from build123d import *

# Parameters (mm, degrees)
F0_R      = 12.805228
F1_DEPTH  = 13.462
F2_R      = 2.775496
F3_DEPTH  = 71.628
F4_DEPTH  = 25.4
F5_DEPTH  = 25.4
F7_DEPTH  = 65.024
F8_R      = 11.544918
F8_R_2    = 5.557541
F8_R_3    = 8.380392
F8_R_4    = 9.320439
F8_R_5    = 10.745749
F8_R_6    = 2.177584
F8_R_7    = 5.592023
F8_R_8    = 5.45278
F8_R_9    = 2.581521
F8_R_10   = 2.292272
F8_R_11   = 6.096395
F8_R_12   = 5.062779
F8_R_13   = 2.606224
F8_R_14   = 5.024667
F8_R_15   = 1.825412
F8_R_16   = 5.73906
F8_R_17   = 5.381808
F8_R_18   = 3.280323
F8_R_19   = 4.310801
F8_R_20   = 2.82533
F8_R_21   = 6.868943
F8_R_22   = 3.579928
F8_R_23   = 2.581522
F8_R_24   = 4.081744
F8_R_25   = 4.869226
F8_R_26   = 2.95209
F8_R_27   = 2.177582
F8_R_28   = 2.726392
F8_R_29   = 1.789965
F8_R_30   = 2.087438
F8_R_31   = 11.06868
F8_R_32   = 2.952267
F9_DEPTH  = 12.954
F10_W     = 19.802404
F10_H     = 13.06525
F10_W_2   = 20.198451
F10_H_2   = 12.933277
F11_DEPTH = 4.064
F13_DEPTH = 5.842


with BuildPart() as f1:
    # F0 (on Right) → F1 (new body)
    with BuildSketch(Plane.YZ):
        Polygon((-62.617041, 14.065981), (-45.4152, 25.146002), (0, 50.444398), (45.4152, 25.146002), (62.617041, 14.065981), (53.866774, 27.880948), (0, 60.095742), (-53.866774, 27.880948), align=None)
        Polygon((0, 50.444398), (-45.4152, 25.146002), (-45.4152, -55.321198), (45.415204, -55.321198), (45.4152, 25.146002), align=None)
        with Locations((0, 6.2484)):
            Circle(F0_R, mode=Mode.SUBTRACT)
    extrude(amount=F1_DEPTH)

    # F2 (on Right) → F3 (join)
    with BuildSketch(Plane.YZ):
        with Locations((0, -32.101408)):
            Circle(F2_R)
    extrude(amount=F3_DEPTH)

    # F0 (on Right) → F4 (join)
    with BuildSketch(Plane.YZ):
        Polygon((-62.617041, 14.065981), (-45.4152, 25.146002), (0, 50.444398), (45.4152, 25.146002), (62.617041, 14.065981), (53.866774, 27.880948), (0, 60.095742), (-53.866774, 27.880948), align=None)
        Polygon((0, 50.444398), (-45.4152, 25.146002), (-45.4152, -55.321198), (45.415204, -55.321198), (45.4152, 25.146002), align=None)
        with Locations((0, 6.2484)):
            Circle(F0_R, mode=Mode.SUBTRACT)
    extrude(amount=F4_DEPTH)

    # F0 (on Right) → F5 (join)
    with BuildSketch(Plane.YZ):
        Polygon((-62.617041, 14.065981), (-45.4152, 25.146002), (0, 50.444398), (45.4152, 25.146002), (62.617041, 14.065981), (53.866774, 27.880948), (0, 60.095742), (-53.866774, 27.880948), align=None)
        Polygon((0, 50.444398), (-45.4152, 25.146002), (-45.4152, -55.321198), (45.415204, -55.321198), (45.4152, 25.146002), align=None)
        with Locations((0, 6.2484)):
            Circle(F0_R, mode=Mode.SUBTRACT)
    extrude(amount=F5_DEPTH)

    # F6 (on face) → F7 (join)
    with BuildSketch(Plane(origin=(0, 0, 0), x_dir=(0, -1, 0), z_dir=(-1, 0, 0))):
        Polygon((53.866774, 27.880948), (0, 60.095742), (-53.866774, 27.880948), (-62.617041, 14.065981), (-45.4152, 25.146002), (-45.415204, -55.321198), (45.4152, -55.321198), (45.4152, 25.146002), (62.617041, 14.065981), align=None)
    extrude(amount=F7_DEPTH)

    # F8 (on face) → F9 (cut)
    with BuildSketch(Plane.XZ.offset(45.4152)):
        with Locations((-47.735427, -38.178124)):
            Circle(F8_R)
        with Locations((-49.167398, -12.04466)):
            Circle(F8_R_2)
        with Locations((-34.489699, -20.636484)):
            Circle(F8_R_3)
        with Locations((-37.353639, 0)):
            Circle(F8_R_4)
        with Locations((13.839315, -7.390756)):
            Circle(F8_R_5)
        with Locations((-16.23207, -18.846521)):
            Circle(F8_R_6)
        with Locations((-26.971854, -35.672177)):
            Circle(F8_R_7)
        with Locations((-3.344336, -22.068456)):
            Circle(F8_R_8)
        with Locations((6.679456, -21.35247)):
            Circle(F8_R_9)
        with Locations((6.321463, -31.376265)):
            Circle(F8_R_10)
        with Locations((16.345263, -30.302286)):
            Circle(F8_R_11)
        with Locations((12.407344, -44.621993)):
            Circle(F8_R_12)
        with Locations((20.641174, -49.63389)):
            Circle(F8_R_13)
        with Locations((-4.060321, -9.180719)):
            Circle(F8_R_14)
        with Locations((-26.613861, -8.106741)):
            Circle(F8_R_15)
        with Locations((-18.022032, -9.896705)):
            Circle(F8_R_16)
        with Locations((-16.590061, 7.644936)):
            Circle(F8_R_17)
        with Locations((0, 9.434899)):
            Circle(F8_R_18)
        with Locations((15.98727, 8.718913)):
            Circle(F8_R_19)
        with Locations((4.173508, 4.423001)):
            Circle(F8_R_6)
        with Locations((-10.86218, 0)):
            Circle(F8_R_20)
        with Locations((-56.327246, 0)):
            Circle(F8_R_21)
        with Locations((-60.623161, -10.254697)):
            Circle(F8_R_22)
        with Locations((-49.167398, -20.994477)):
            Circle(F8_R_23)
        with Locations((-57.759218, -19.562507)):
            Circle(F8_R_24)
        with Locations((-31.267766, -45.695972)):
            Circle(F8_R_25)
        with Locations((-19.812003, -26.006375)):
            Circle(F8_R_26)
        with Locations((-24.107913, -51.781844)):
            Circle(F8_R_27)
        with Locations((-60.623161, -47.12794)):
            Circle(F8_R_28)
        with Locations((-62.413126, -27.796337)):
            Circle(F8_R_29)
        with Locations((-39.501593, -50.349873)):
            Circle(F8_R_30)
        with Locations((-9.707933, -40.136304)):
            Circle(F8_R_31)
        with Locations((2.335547, -49.885787)):
            Circle(F8_R_32)
    extrude(amount=-F9_DEPTH, mode=Mode.SUBTRACT)

    # F10 (on face) → F11 (join)
    with BuildSketch(Plane(origin=(0, 45.415201, 2e-06), x_dir=(-1, 0, 0), z_dir=(0, 1, 0))):
        Polygon((41.411106, -3.204356), (-7.916423, -3.578231), (-7.916423, -37.325934), (41.411106, -37.325934), align=None)
        Polygon((-5.569554, -34.437824), (-5.569554, -22.560325), (-5.569554, -21.900464), (14.496882, -21.900464), (14.496882, -23.220185), (14.496882, -34.437824), (13.572769, -34.437824), align=None, mode=Mode.SUBTRACT)
        Polygon((17.929297, -34.701772), (17.929297, -21.504547), (37.7317, -21.768492), (37.7317, -34.701772), align=None, mode=Mode.SUBTRACT)
        with Locations((4.331648, -12.992339)):
            Rectangle(F10_W, F10_H, mode=Mode.SUBTRACT)
        with Locations((28.292554, -12.926353)):
            Rectangle(F10_W_2, F10_H_2, mode=Mode.SUBTRACT)
    extrude(amount=F11_DEPTH)

    # F12 (on face) → F13 (join)
    with BuildSketch(Plane(origin=(-65.024, 0, 0), x_dir=(0, -1, 0), z_dir=(-1, 0, 0))):
        Polygon((-43.786074, -20.438465), (2.748472, 0), (-38.219031, 30.080867), align=None)
        Polygon((3.604237, -53.453038), (3.604237, -3.573573), (-39.592647, -28.513306), align=None)
        Polygon((22.778634, -18.640616), (11.063425, -50.157975), (44.215863, -44.544963), align=None)
        Polygon((9.034589, -19.765744), (38.46338, -0.555568), (7.112485, 15.325424), align=None)
        Polygon((0, 56.749567), (-10.859401, 15.269949), (30.492702, 26.605241), align=None)
    extrude(amount=F13_DEPTH)


solid = f1.part
The model under review builds one solid part; all positions refer to its coordinate system, in mm. A direction names the side the tool comes from. Round coordinates to 2 decimals unless told otherwise and drop trailing zeros. Loops run counter-clockwise (first coordinate to the right, second up) from the corner with the lowest first, then second, coordinate; pieces in that order, holes last. Notation, with made-up numbers: M 46,19.25 L 65,19.25 A14 ccw 65,30.25 Z; hole C 7,-7 d6. An arc over 180 degrees is marked long. Answer as CSV lines item,"result".
1. For faces 4 (the face through (-61, -32.461, -10)), 5 (the face through (-19.18, -58.3, 20.88)), 6 (the face through (12.52, -2.78, -6.25)), 7 (the face through (5.57, 47, -13)), list the 3-axis set-ups (+Z, -Z, +X, -X, +Y, -Y) from which the entire face can be reached by the end or side of a thin tool; tool diameter is ignored.
Outcome:
face 4,"-Y"
face 5,"+Z, +X, -X, -Y"
face 6,"+X"
face 7,"+Y"
2. We need section A-A (z = 49). Give the boundary of the cut face in (x, y).
Outcome:
outline,"M -70.87,-7.84 L -65.02,-7.84 L -65.02,-18.55 L 25.4,-18.55 L 25.4,18.55 L -65.02,18.55 L -65.02,2.03 L -70.87,2.03 Z"
3. Draft analysis for pull direction X (two halves, no side actions). For faces 1 (the face through (-28, 47, -6.46)), 2 (the face through (-19, -45.415, -16)), 3 (the face through (71.628, 0, -32)), state which applies: pulls with the +X half, pulls with the -X half, needs draft (parallel to the pull), parting line crosses it, or undercut.
Outcome:
face 1,"undercut"
face 2,"needs draft"
face 3,"pulls with the +X half"
4. To check wall thickness, follow L1, parallel to X at y = -42, z = -12; L2, parallel to Y at x = 3.5, z = 16; L3, parallel to X at y = 7.5, z = 38. State the ranges of each line that lie inside material, in increasing order. Write a range as [from, to].
Outcome:
L1,"x = [-65.02, -63.75], [-57.5, -54.72], [-43.61, -23.36], [-12.68, -8.22], [0.1, 4.13], [23.55, 25.4]"
L2,"y = [-61.39, -59.61], [-45.42, -8.3], [8.3, 45.42], [59.61, 61.39]"
L3,"x = [-65.02, 25.4]"
5. We need section D-D (z = 32). Give the boundary of the cut face in (x, y).
Outcome:
outline,"M -70.87,-25.04 L -65.02,-25.04 L -65.02,-46.98 L 25.4,-46.98 L 25.4,46.98 L -65.02,46.98 L -65.02,6.48 L -70.87,6.48 Z"
6. We need section B-B (x = 50). Give the boundary of the cut face in (y, z), plus the area to 3 significant figures.
Outcome:
outline,"C 0,-32.1 d5.55"
area,"24.2 mm2"
7. Insertion check: pin 1 Ø6.5 at (x, z) = (-3.34, -22.07) entering from +Y; pin 2 Ø1.3 at (x, z) = (-40, -50) entering from -Y; pin 3 Ø6 at (x, z) = (-27, 15.5) entering from -Y. Each pin has a flat end and moves straight along its axis. Give the tip position at first contact, or say it passes through.
Outcome:
pin 1,"stops at y = 49.48"
pin 2,"stops at y = -32.46"
pin 3,"stops at y = -62.62"
8. We need section C-C (y = 52). Give the boundary of the cut face in (x, z), plus the area to 3 significant figures.
Outcome:
outline,"M -65.02,20.9 L 25.4,20.9 L 25.4,29 L -65.02,29 Z"
area,"732 mm2"
